The model under review builds one solid part; all positions refer to its coordinate system, in mm. A direction names the side the tool comes from. Coordinates: 2 decimals unless noted, no trailing zeros. Loops run counter-clockwise (first coordinate to the right, second up) from the corner with the lowest first, then second, coordinate; pieces in that order, holes last. Notation, with made-up numbers: (76, 52.25) - (82, 52.25) arc R21 ccw to (82, 59.25) - close; hole circle Ø9 at (-7.75, -18.5). An arc over 180 degrees is marked (long way). Answer in a Markdown table with one row per item. Add a question column.
(1) Machinability: for faces 4 (the flat face through (-5, -2, 25)), 5 (the cylindrical face through (-54, -2.43, 42.29)), 6 (the flat face through (-50, -2, 20)), 7 (the flat face through (-53, -3, 5.5)), which of the approach directions +Z, -Z, +X, -X, +Y, -Y give a long, thin tool a straight path to every point of the face, cutting with its end or side? Answer none if there is none.
(2) For P1, Ø2.5, axis at x = -53, y = -2.5, coming from the -Z side; P2, Ø2.5, axis at x = -52.5, y = -2.5, coming from the +Z side; P3, Ø2.5, axis at x = -2.5, y = -2.5, coming from the -Z side, all flat-tipped, find the tip position at first contact; note any pin that passes through.
(3) Mouldability with a two-part tool opening along Y and no side actions: class faces 1 (the flat face through (-28, 0, 24)), 2 (the flat face through (-4.3, -2.5, 0)), 3 (the cylindrical face through (-1.81, -1.17, 2.71)) as +Y half, -Y half, draft (parallel to the pull), parting line (faces both ways), or undercut.
(4) We need section D-D on x = -52.5. Write out the cut boundary in (y, z), plus the area to 3 significant figures.
(5) We need section A-A on z = 36.5. Write out the cut boundary in (x, y), plus the area to 3 significant figures.
(6) For line 1 along X through (y, z) = (-1.65, 9.5); line 2 along X through (y, z) = (-4.6, 14); line 3 along Y through (x, z) = (-2.5, 41.05), list the stretches that pass through material, from the lowest coordinate up.
(7) We need section C-C on y = -2.5. Write out the cut boundary in (x, z), plus the area to 3 significant figures.
(8) We need section B-B on z = 4.5. Write out the cut boundary in (x, y).
from build123d import *

# Parameters (mm, degrees)
F1_DEPTH = 5
F2_R     = 1.5
F2_R_2   = 4.115786
F3_DEPTH = 5.5
F4_R     = 1.5
F5_DEPTH = 5.5


with BuildPart() as f1:
    # F0 (on Front) → F1 (new body)
    with BuildSketch(Plane.XZ):
        Polygon((-46.464466, 45), (-55, 45), (-55, 0), (-50, 0), (-50, 41.464466), (-8.535534, 0), (0, 0), (0, 45), (-5, 45), (-5, 3.535534), align=None)
    extrude(amount=F1_DEPTH)

    # F2 (on face) → F3 (cut)
    with BuildSketch(Plane.XY.offset(45)):
        with Locations((-52.5, -2.5)):
            Circle(F2_R)
        with Locations((-2.5, -2.5)):
            Circle(F2_R)
        with Locations((101.68349, -24.659157)):
            Circle(F2_R_2)
    extrude(amount=-F3_DEPTH, mode=Mode.SUBTRACT)

    # F4 (on face) → F5 (cut)
    with BuildSketch(Plane(origin=(0, 0, 0), x_dir=(1, 0, 0), z_dir=(0, 0, -1))):
        with Locations((-52.5, 2.5)):
            Circle(F4_R)
        with Locations((-2.5, 2.5)):
            Circle(F4_R)
    extrude(amount=-F5_DEPTH, mode=Mode.SUBTRACT)


solid = f1.part
Outcome:
| question | item | result |
|---|---|---|
| 1 | face 4 | +Z, +Y, -Y |
| 1 | face 5 | +Z |
| 1 | face 6 | -Z, +Y, -Y |
| 1 | face 7 | -Z |
| 2 | P1 | z = 0 |
| 2 | P2 | z = 39.5 |
| 2 | P3 | z = 5.5 |
| 3 | face 1 | +Y half |
| 3 | face 2 | draft |
| 3 | face 3 | undercut |
| 4 | outline | (-5, 0) - (-4, 0) - (-4, 5.5) - (-1, 5.5) - (-1, 0) - (0, 0) - (0, 45) - (-1, 45) - (-1, 39.5) - (-4, 39.5) - (-4, 45) - (-5, 45) - close |
| 4 | area | 192 mm² |
| 5 | outline | (-55, -5) - (-50, -5) - (-50, 0) - (-55, 0) - close; (-45.04, -5) - (-37.96, -5) - (-37.96, 0) - (-45.04, 0) - close; (-5, -5) - (0, -5) - (0, 0) - (-5, 0) - close |
| 5 | area | 85.4 mm² |
| 6 | line 1 | -55 to -50, -18.04 to -10.96, -5 to 0 |
| 6 | line 2 | -55 to -50, -22.54 to -15.46, -5 to 0 |
| 6 | line 3 | -5 to -4, -1 to 0 |
| 7 | outline | (-55, 0) - (-54, 0) - (-54, 5.5) - (-51, 5.5) - (-51, 0) - (-50, 0) - (-50, 41.46) - (-8.54, 0) - (-4, 0) - (-4, 5.5) - (-1, 5.5) - (-1, 0) - (0, 0) - (0, 45) - (-1, 45) - (-1, 39.5) - (-4, 39.5) - (-4, 45) - (-5, 45) - (-5, 3.54) - (-46.46, 45) - (-51, 45) - (-51, 39.5) - (-54, 39.5) - (-54, 45) - (-55, 45) - close |
| 7 | area | 690 mm² |
| 8 | outline | (-55, -5) - (-50, -5) - (-50, 0) - (-55, 0) - close; (-13.04, -5) - (-5.96, -5) - (-5.96, 0) - (-13.04, 0) - close; (-5, -5) - (0, -5) - (0, 0) - (-5, 0) - close; hole circle Ø3 at (-52.5, -2.5); hole circle Ø3 at (-2.5, -2.5) |
